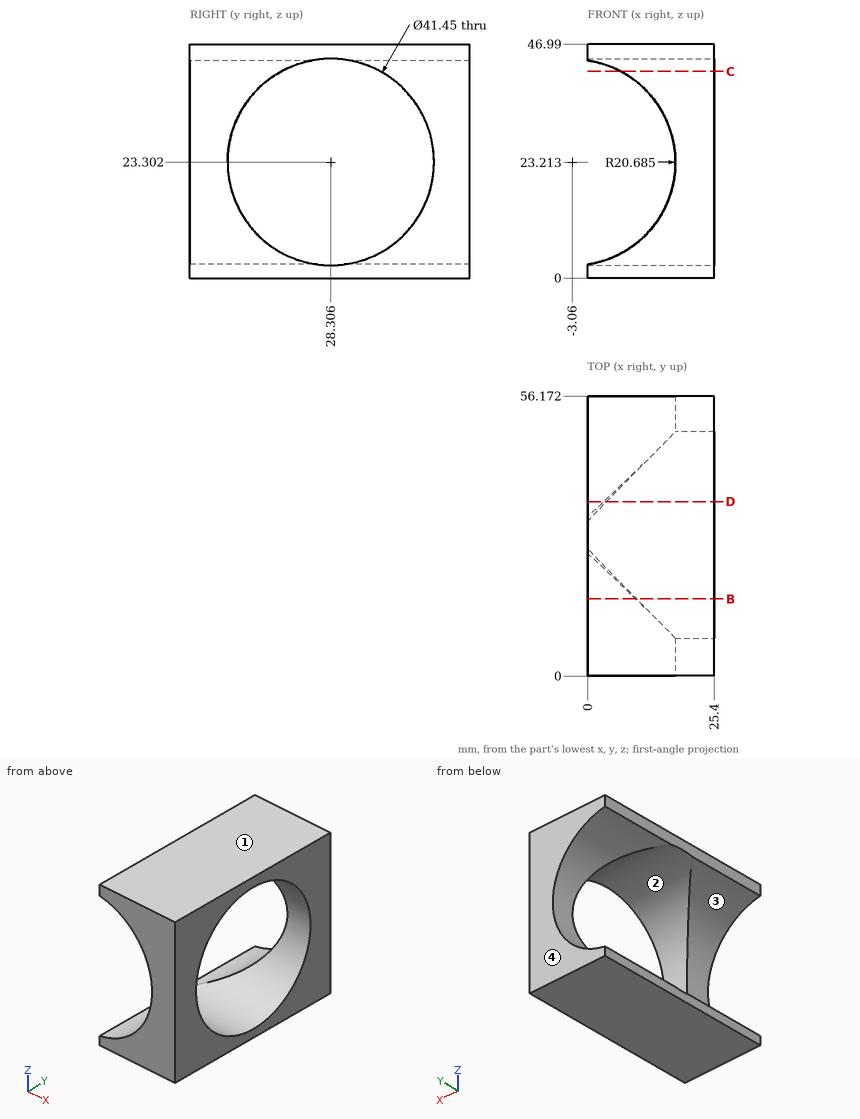
Can you work these out from the drawing? Everything is in mm from the part's minimum corner. Round coordinates to 2 decimals unless told otherwise and drop trailing zeros. Loops run counter-clockwise (first coordinate to the right, second up) from the corner with the lowest first, then second, coordinate; pieces in that order, holes last.
1. If I drill on line 1 along Z through (x, y) = (24, 10) (1 decimal); line 2 along Z through (x, y) = (7, 53.5); line 3 along Y through (x, z) = (21.25, 30), over which ranges is the centre line in solid material (lowest first)?
Answer list:
line 1: z = 0 to 13.6, 33 to 47
line 2: z = 0 to 5.14, 41.29 to 46.99
line 3: y = 0 to 8.69, 47.92 to 56.17
2. If we section it at C-C on z = 41.5: Write out the boundary of the cut face in (x, y), plus the area to 3 significant figures.
Answer list:
outline: (6.61, 0) - (25.4, 0) - (25.4, 18.39) - (6.61, 18.39) - close; (6.61, 38.22) - (25.4, 38.22) - (25.4, 56.17) - (6.61, 56.17) - close
area: 683 mm2
3. If we section it at D-D on y = 35: Write out the boundary of the cut face in (x, z) (1 decimal).
Answer list:
outline: (0, 0) - (25.4, 0) - (25.4, 3.7) - (3.8, 3.7) arc R20.7 cw to (0, 2.8) - close; (0, 43.7) arc R20.7 cw to (3.2, 42.9) - (25.4, 42.9) - (25.4, 47) - (0, 47) - close
4. If we section it at B-B on y = 15.5: Write out the boundary of the cut face in (x, z) (1 decimal).
Answer list:
outline: (0, 0) - (25.4, 0) - (25.4, 7) - (9.8, 7) arc R20.7 cw to (0, 2.8) - close; (0, 43.7) arc R20.7 cw to (9.6, 39.6) - (25.4, 39.6) - (25.4, 47) - (0, 47) - close
5. For P1, Ø12, axis at y = 45, z = 22.5, coming from the -X side; P2, Ø4, axis at y = 48.5, z = 7, coming from the -X side (1 decimal), each with a flat end and sliding along its axis, tell me the tip position at first contact or that it passes through.
Answer list:
P1: stops at x = 16.79
P2: stops at x = 6.7
6. We'd pull the mould along Z, two halves only. Please class the marked faces 1, 2, 3 and 4: +Z half, -Z half, draft (parallel to the pull), parting line (faces both ways), or undercut.
Answer list:
face 1: +Z half
face 2: undercut
face 3: undercut
face 4: draft
